Model file for the job. Use its own axes, mm. A direction names the side the tool comes from. Give positions to 0.01 mm unless a question says otherwise; leave off trailing zeros. Write each loop counter-clockwise with the first axis right and the second up, starting at its lowest first coordinate (ties: lowest second). Pieces come first, ordered by that corner, then holes.
```python
from build123d import *

# Parameters (mm, degrees)
IRON_V40X40X3_1_DEPTH = 260
CUT_EXTRUDE1_DEPTH    = 10


with BuildPart() as part:
    # Sketch1 → Iron V40X40X3(1) (new body)
    with BuildSketch(Plane(origin=(0, 0, 0), x_dir=(1, 0, 0), z_dir=(0, 1, 0))):
        with BuildLine():
            Line((0, 0), (0, 40))
            ThreePointArc((0, 40), (2.121320344, 39.121320344), (3, 37))
            Line((3, 37), (3, 6.5))
            ThreePointArc((3, 6.5), (4.025126266, 4.025126266), (6.5, 3))
            Line((6.5, 3), (37, 3))
            ThreePointArc((37, 3), (39.121320344, 2.121320344), (40, 0))
            Line((40, 0), (0, 0))
        make_face()
    extrude(amount=IRON_V40X40X3_1_DEPTH)

    # Sketch2 → Cut-Extrude1 (cut)
    with BuildSketch(Plane.XY):
        with BuildLine():
            Line((10.5, 55), (25.5, 55))
            ThreePointArc((25.5, 55), (30.5, 50), (25.5, 45))
            Line((25.5, 45), (10.5, 45))
            ThreePointArc((10.5, 45), (5.5, 50), (10.5, 55))
        make_face()
        with BuildLine():
            Line((10.5, 85), (25.5, 85))
            ThreePointArc((25.5, 85), (30.5, 80), (25.5, 75))
            Line((25.5, 75), (10.5, 75))
            ThreePointArc((10.5, 75), (5.5, 80), (10.5, 85))
        make_face()
        with BuildLine():
            Line((10.5, 205), (25.5, 205))
            ThreePointArc((25.5, 205), (30.5, 200), (25.5, 195))
            Line((25.5, 195), (10.5, 195))
            ThreePointArc((10.5, 195), (5.5, 200), (10.5, 205))
        make_face()
        with BuildLine():
            Line((10.5, 235), (25.5, 235))
            ThreePointArc((25.5, 235), (30.5, 230), (25.5, 225))
            Line((25.5, 225), (10.5, 225))
            ThreePointArc((10.5, 225), (5.5, 230), (10.5, 235))
        make_face()
    extrude(amount=-CUT_EXTRUDE1_DEPTH, mode=Mode.SUBTRACT)


solid = part.part
```
1. Probe probe 1 along X at (y, z) = (182.5, -6); probe 2 along Z at (x, y) = (19.5, 23.5); probe 3 along Z at (x, y) = (5, 105). List the from-to ranges inside material, lowest first.
Calculated:
probe 1: x = 0 to 3.04
probe 2: z = -3 to 0
probe 3: z = -3.34 to 0
2. Slice it at B-B, the plane y = 230. Write the cut outline in (x, z), and give its area (3 significant figures).
Calculated:
outline: (0, -40) arc R3 ccw to (3, -37) - (3, -6.5) arc R3.5 cw to (5.5, -3.15) - (5.5, 0) - (0, 0) - close; (30.5, -3) - (37, -3) arc R3 ccw to (40, 0) - (30.5, 0) - close
area: 155 mm2
3. Pull direction X, two halves, no side cores. Call faces 1 (the cylindrical face through (5.5, 49.9, -1.6)), 2 (the cylindrical face through (30.5, 80.1, -1.5)), 3 (the flat face through (0, 128, -20)), 4 (the flat face through (11, 0, -2)): +X half, -X half, draft (parallel to the pull), parting line (faces both ways), or undercut.
Calculated:
face 1: undercut
face 2: undercut
face 3: -X half
face 4: draft
4. Which spindle directions (+Z, -Z, +X, -X, +Y, -Y) get a long thin tool onto all of the face, cutting with end or side? Do faces 5 (the cylindrical face through (5.5, 199.9, -1.6)), 6 (the flat face through (22, 128, -3)), 7 (the flat face through (20, 128, 0)). Say none if no direction does.
Calculated:
face 5: +Z, -Z
face 6: -Z, +X, +Y, -Y
face 7: +Z, +X, -X, +Y, -Y
5. Slice it at A-A, the plane x = 20.5. Write the cut outline in (y, z), and give its area (3 significant figures).
Calculated:
outline: (0, -3) - (45, -3) - (45, 0) - (0, 0) - close; (55, -3) - (75, -3) - (75, 0) - (55, 0) - close; (85, -3) - (195, -3) - (195, 0) - (85, 0) - close; (205, -3) - (225, -3) - (225, 0) - (205, 0) - close; (235, -3) - (260, -3) - (260, 0) - (235, 0) - close
area: 660 mm2
6. Pin check, flat tips, straight feed: P1, Ø4, axis at y = 81, z = -24.5, coming from the +X side; P2, Ø10, axis at x = 24.5, y = 59, coming from the -Z side. Stop position of each tip, or through.
Calculated:
P1: stops at x = 3
P2: stops at z = -3
